Read the model definition and answer for the solid it produces. Units are mm, in the model's axes. A direction names the side the tool comes from. Coordinates: 2 decimals unless noted, no trailing zeros. Loops run counter-clockwise (first coordinate to the right, second up) from the corner with the lowest first, then second, coordinate; pieces in that order, holes last. Notation, with made-up numbers: (-18, 59) -> (-7, 59) arc R27 cw to (-7, 87) -> close; hole circle Ø9 at (-29, 42). An arc over 180 degrees is marked (long way). Answer as CSV lines item,"result".
```python
from build123d import *

# Parameters (mm, degrees)
BASE_FLANGE1_DEPTH = 6
HEM1_START         = 50
HEM1_DEPTH         = 200
HEM1_2_DEPTH       = 50
HEM1_START_2       = 200
HEM1_3_DEPTH       = 50
SKETCH11_R         = 15
CUT_EXTRUDE1_DEPTH = 10


# Read off the part's stored shape, not the designer's step: Hem1
# Sheet-metal steps are written as plain solids
with BuildPart() as part:
    # Sketch2 → Base-Flange1 (new body)
    with BuildSketch(Plane.XY):
        with BuildLine():
            Line((20, 0), (280, 0))
            ThreePointArc((280, 0), (294.142135624, 5.857864376), (300, 20))
            Line((300, 20), (300, 115))
            Line((300, 115), (250, 115))
            Line((250, 115), (250, 165))
            Line((250, 165), (200, 165))
            Line((200, 165), (200, 115))
            Line((200, 115), (100, 115))
            Line((100, 115), (100, 165))
            Line((100, 165), (50, 165))
            Line((50, 165), (50, 115))
            Line((50, 115), (0, 115))
            Line((0, 115), (0, 20))
            ThreePointArc((0, 20), (5.857864376, 5.857864376), (20, 0))
        make_face()
    extrude(amount=-BASE_FLANGE1_DEPTH)

    # Hem1 outline → Hem1 (cut)
    with BuildSketch(Plane.YZ.offset(HEM1_START)):
        with BuildLine():
            Line((165, 0), (162.95445115, 0))
            ThreePointArc((162.95445115, 0), (158.244997998, -4.401754251), (152, -6))
            Line((152, -6), (165, -6))
            Line((165, -6), (165, 0))
        make_face()
    extrude(amount=HEM1_DEPTH, mode=Mode.SUBTRACT)

    # Hem1 2 outline → Hem1 2 (add)
    with BuildSketch(Plane.YZ.offset(HEM1_START)):
        with BuildLine():
            Line((120.297159916, 5.436837245), (123.021102914, 0.0907981))
            Line((123.021102914, 0.0907981), (148.822066502, 13.237045669))
            ThreePointArc((148.822066502, 13.237045669), (158.806589443, 8.634117547), (152, 0))
            Line((152, 0), (162.95445115, 0))
            ThreePointArc((162.95445115, 0), (161.628857043, 15.734134876), (146.098123503, 18.583084814))
            Line((146.098123503, 18.583084814), (120.297159916, 5.436837245))
        make_face()
    extrude(amount=HEM1_2_DEPTH)

    # Hem1 3 outline → Hem1 3 (add)
    with BuildSketch(Plane.YZ.offset(HEM1_START_2)):
        with BuildLine():
            Line((120.297159916, 5.436837245), (123.021102914, 0.0907981))
            Line((123.021102914, 0.0907981), (148.822066502, 13.237045669))
            ThreePointArc((148.822066502, 13.237045669), (158.806589443, 8.634117547), (152, 0))
            Line((152, 0), (162.95445115, 0))
            ThreePointArc((162.95445115, 0), (161.628857043, 15.734134876), (146.098123503, 18.583084814))
            Line((146.098123503, 18.583084814), (120.297159916, 5.436837245))
        make_face()
    extrude(amount=HEM1_3_DEPTH)

    # Sketch11 → Cut-Extrude1 (cut)
    with BuildSketch(Plane.XY):
        with Locations((250, 60)):
            Circle(SKETCH11_R)
        with Locations((150, 60)):
            Circle(SKETCH11_R)
        with Locations((50, 60)):
            Circle(SKETCH11_R)
    extrude(amount=-CUT_EXTRUDE1_DEPTH, mode=Mode.SUBTRACT)


solid = part.part
```
Q1. For a pull along Z with two mould halves and no side action, classify faces 1 (the face through (148, 77, -6)), 2 (the face through (224.65, 121.64, 2.8)), 3 (the face through (300, 67, -3)) as pulls with the +Z half, pulls with the -Z half, needs draft (parallel to the pull), parting line crosses it, or undercut.
Results:
face 1,"pulls with the -Z half"
face 2,"undercut"
face 3,"needs draft"
Q2. A cutting plane is placed at A-A, the plane x = 150. Write down the section's boundary in (y, z), and give its area (3 significant figures).
Results:
outline,"(0, -6) -> (45, -6) -> (45, 0) -> (0, 0) -> close; (75, -6) -> (115, -6) -> (115, 0) -> (75, 0) -> close"
area,"510 mm²"
Q3. Find the intervals of material crossed by probe 1 along X at (y, z) = (147.5, 15.75); probe 2 along Z at (x, y) = (72, 152); probe 3 along Y at (x, z) = (150, -4.05), in increasing order. Write a range as [from, to].
Results:
probe 1,"x = [50, 100], [200, 250]"
probe 2,"z = [-6, 0], [14, 20]"
probe 3,"y = [0, 45], [75, 115]"
Q4. A cutting plane is placed at C-C, the plane y = 83.5. Write down the section's boundary in (x, z).
Results:
outline,"(0, -6) -> (300, -6) -> (300, 0) -> (0, 0) -> close"
Q5. Given pin 1 Ø1.5 at (x, z) = (105.5, -2.5) entering from +Y; pin 2 Ø10 at (x, y) = (90.5, 38.5) entering from +Z; pin 3 Ø5 at (y, z) = (144.5, 17.5) entering from +X, each flat-ended and moving along its own axis, determine where each tip first touches the part or whether it passes through.
Results:
pin 1,"stops at y = 115"
pin 2,"stops at z = 0"
pin 3,"stops at x = 250"
Q6. A cutting plane is placed at D-D, the plane x = 44. Write down the section's boundary in (y, z), and give its area (3 significant figures).
Results:
outline,"(0, -6) -> (46.25, -6) -> (46.25, 0) -> (0, 0) -> close; (73.75, -6) -> (115, -6) -> (115, 0) -> (73.75, 0) -> close"
area,"525 mm²"
Q7. A cutting plane is placed at B-B, the plane z = 8.5. Write down the section's boundary in (x, y).
Results:
outline,"(50, 126.31) -> (100, 126.31) -> (100, 139.53) -> (50, 139.53) -> close; (50, 158.84) -> (100, 158.84) -> (100, 164.91) -> (50, 164.91) -> close; (200, 126.31) -> (250, 126.31) -> (250, 139.53) -> (200, 139.53) -> close; (200, 158.84) -> (250, 158.84) -> (250, 164.91) -> (200, 164.91) -> close"
Q8. For faces 4 (the face through (250, 140, -1)), 5 (the face through (74.65, 121.64, 2.8)), 6 (the face through (200, 140, -1)), 7 (the face through (50, 140, -1)), determine the directions among +Z, -Z, +X, -X, +Y, -Y from which every point of the face is accessible in a straight line to the end or side of a thin tool.
Results:
face 4,"+Z, -Z, +X, +Y"
face 5,"+X, -X, -Y"
face 6,"+Z, -Z, +Y"
face 7,"+Z, -Z, -X, +Y"
